from build123d import *

# Parameters (mm, degrees)
CROQUIS1_R              = 5
CROQUIS1_R_2            = 6.417351574
SALIENTE_EXTRUIR1_DEPTH = 5


with BuildPart() as part:
    # Croquis1 → Saliente-Extruir1 (new body)
    with BuildSketch(Plane.XY):
        with BuildLine():
            Line((-70, 10), (68.594591653, 10))
            Line((68.594591653, 10), (116.267972935, 23.670122106))
            ThreePointArc((116.267972935, 23.670122106), (128.636963452, 16.813878705), (121.780720051, 4.444888187))
            Line((121.780720051, 4.444888187), (72.756373558, -9.612616959))
            ThreePointArc((72.756373558, -9.612616959), (71.39173101, -9.902680687), (70, -10))
            Line((70, -10), (-70, -10))
            ThreePointArc((-70, -10), (-80, 0), (-70, 10))
        make_face()
        with Locations((70, 0)):
            Circle(CROQUIS1_R, mode=Mode.SUBTRACT)
        with Locations((119.024346493, 14.057505147)):
            Circle(CROQUIS1_R, mode=Mode.SUBTRACT)
        with Locations((-70, 0)):
            Circle(CROQUIS1_R_2, mode=Mode.SUBTRACT)
    extrude(amount=SALIENTE_EXTRUIR1_DEPTH)


solid = part.part
Verification items for the finished model (mm, model axes). Round coordinates to 2 decimals unless told otherwise and drop trailing zeros. Write each loop counter-clockwise with the first axis right and the second up, starting at its lowest first coordinate (ties: lowest second). Pieces come first, ordered by that corner, then holes.
(1) Section check A-A (y = 0). Enter the section's corners in (x, z).
Returned:
outline: (-80, 0) - (-76.42, 0) - (-76.42, 5) - (-80, 5) - close; (-63.58, 0) - (65, 0) - (65, 5) - (-63.58, 5) - close; (75, 0) - (106.28, 0) - (106.28, 5) - (75, 5) - close
(2) Material ranges on line 1 (Y direction, x = -70, z = 3.3); line 2 (Y direction, x = 70, z = 3.4); line 3 (Y direction, x = -41.5, z = 2.2), recorded low to high.
Returned:
line 1: y = -10 to -6.42, 6.42 to 10
line 2: y = -10 to -5, 5 to 10.4
line 3: y = -10 to 10
(3) Mould release check, pull along Y, two halves, no side actions. Record for faces 1 (the flat face through (26, 3, 0)), 2 (the cylindrical face through (74.619, -1.915, 2.465)), 3 (the cylindrical face through (123.793, 15.559, 2.465)), 4 (the flat face through (-2, 10, 2)): pulls with the +Y half, pulls with the -Y half, needs draft (parallel to the pull), parting line crosses it, or undercut.
Returned:
face 1: needs draft
face 2: undercut
face 3: undercut
face 4: pulls with the +Y half
(4) Depth check by flat-ended pin: pin 1 Ø7.5 at (x, y) = (-70, 0) entering from -Z; pin 2 Ø2 at (y, z) = (5.5, 3.5) entering from +X; pin 3 Ø1 at (y, z) = (7, 3.5) entering from +X; pin 4 Ø2 at (x, z) = (73, 2.5) entering from -Y. Enter the tip coordinate at first touch or a pass-through.
Returned:
pin 1: passes through
pin 2: stops at x = 125.57
pin 3: stops at x = 126.57
pin 4: stops at y = -9.8
(5) Section check B-B (z = 3.05). Enter the section's corners in (x, y), plus the area to 3 significant figures.
Returned:
outline: (-70, -10) - (70, -10) arc R10 ccw to (72.76, -9.61) - (121.78, 4.44) arc R10 ccw to (116.27, 23.67) - (68.59, 10) - (-70, 10) arc R10 ccw to start; hole circle Ø12.83 at (-70, 0); hole circle Ø10 at (70, 0); hole circle Ø10 at (119.02, 14.06)
area: 3,850 mm2
(6) Section check C-C (y = 16). Enter the section's corners in (x, z).
Returned:
outline: (89.52, 0) - (114.42, 0) - (114.42, 5) - (89.52, 5) - close; (123.63, 0) - (128.83, 0) - (128.83, 5) - (123.63, 5) - close
(7) Section check D-D (x = 47.5). Enter the section's corners in (y, z).
Returned:
outline: (-10, 0) - (10, 0) - (10, 5) - (-10, 5) - close
